Source: CAD feature listing. Evaluate the final solid. Frame: model axes, mm. Face numbers are marked on the shaded views. Give positions to 0.01 mm unless a question says otherwise; leave off trailing zeros. Loops run counter-clockwise (first coordinate to the right, second up) from the corner with the lowest first, then second, coordinate; pieces in that order, holes last. Notation, with made-up numbers: (5.25, 43.5) -> (62.25, 43.5) arc R16 cw to (62.25, 54.5) -> close; hole circle Ø10 at (82, 77). An arc over 180 degrees is marked (long way). Return JSON: item names as keys, results as strings. Group by question number.
(1) Pin query (flat end, axial travel): pin 1 (10 mm diameter, centred on x = 5.5, y = 67, fed in from -Z); pin 2 (4 mm diameter, centred on x = 5.5, y = 5.58, fed in from +Z); pin 3 (5 mm diameter, centred on x = 11, y = 56.8, fed in from +Z). Return the tip coordinate at first contact, or that it passes through.
(2) Draft query along X for the marked faces 1, 2 and 3. Return one class per face: released by +X, released by -X, zero draft, split by the parting line, or undercut.
(3) Ray query, line 1 (Y direction, x = 31, z = 4); line 2 (X direction, y = 56.8, z = 1.3); line 3 (Y direction, x = 31, z = 1). Return the intervals inside material, ascending. Write a range as from..to.
(4) Cut plane D-D on z = 4.2. Give the number of separate pieces and of enclosed holes in the cut face, then the cut area to 3 significant figures.
(5) Cut plane C-C on x = 11. Return loops of the section in (y, z).
(6) Cut plane B-B on y = 21.08. Return loops of the section in (x, z), then the cut area to 3 significant figures.
(7) Cut plane A-A on y = 36.58. Return loops of the section in (x, z) (3 decimals), then the cut area to 3 significant figures.
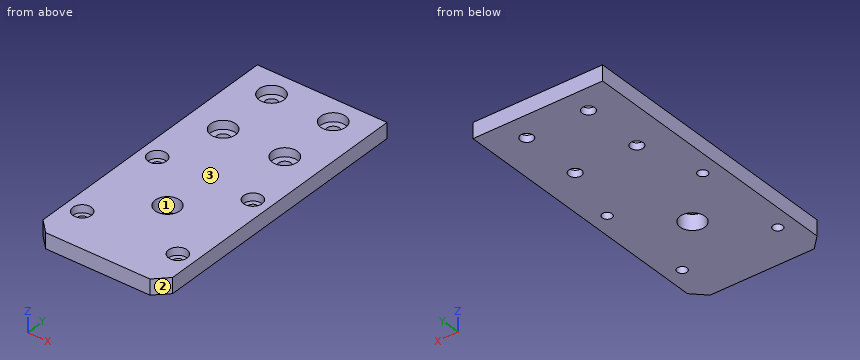
```python
from build123d import *

# Parameters (mm, degrees)
CROQUIS1_W              = 42
CROQUIS1_H              = 85
CROQUIS1_R              = 2.05
SALIENTE_EXTRUIR1_DEPTH = 5
CROQUIS4_R              = 4.05
CORTAR_EXTRUIR1_DEPTH   = 2.8
CROQUIS5_R              = 1.575
CROQUIS5_R_2            = 4
CORTAR_EXTRUIR2_DEPTH   = 6
CROQUIS6_R              = 3
CORTAR_EXTRUIR3_DEPTH   = 2.5
CROQUIS7_W              = 42
CROQUIS7_H              = 7.7
SALIENTE_EXTRUIR2_DEPTH = 5
CHAFL_N1_SIZE           = 4.1


with BuildPart() as part:
    # Croquis1 → Saliente-Extruir1 (new body)
    with BuildSketch(Plane.XY):
        with Locations((21, 42.5)):
            Rectangle(CROQUIS1_W, CROQUIS1_H)
        with Locations((11, 76.8)):
            Circle(CROQUIS1_R, mode=Mode.SUBTRACT)
        with Locations((31, 76.8)):
            Circle(CROQUIS1_R, mode=Mode.SUBTRACT)
        with Locations((31, 56.8)):
            Circle(CROQUIS1_R, mode=Mode.SUBTRACT)
        with Locations((11, 56.8)):
            Circle(CROQUIS1_R, mode=Mode.SUBTRACT)
    extrude(amount=SALIENTE_EXTRUIR1_DEPTH)

    # Croquis4 → Cortar-Extruir1 (cut)
    with BuildSketch(Plane.XY.offset(5)):
        with Locations((11, 76.8)):
            Circle(CROQUIS4_R)
        with Locations((11, 56.8)):
            Circle(CROQUIS4_R)
        with Locations((31, 56.8)):
            Circle(CROQUIS4_R)
        with Locations((31, 76.8)):
            Circle(CROQUIS4_R)
    extrude(amount=-CORTAR_EXTRUIR1_DEPTH, mode=Mode.SUBTRACT)

    # Croquis5 → Cortar-Extruir2 (cut, through all)
    with BuildSketch(Plane.XY.offset(5)):
        with Locations((5.5, 36.58)):
            Circle(CROQUIS5_R)
        with Locations((36.5, 36.58)):
            Circle(CROQUIS5_R)
        with Locations((36.5, 5.58)):
            Circle(CROQUIS5_R)
        with Locations((5.5, 5.58)):
            Circle(CROQUIS5_R)
        with Locations((21, 21.08)):
            Circle(CROQUIS5_R_2)
    extrude(amount=-CORTAR_EXTRUIR2_DEPTH, mode=Mode.SUBTRACT)

    # Croquis6 → Cortar-Extruir3 (cut)
    with BuildSketch(Plane.XY.offset(5)):
        with Locations((5.5, 36.58)):
            Circle(CROQUIS6_R)
        with Locations((36.5, 36.58)):
            Circle(CROQUIS6_R)
        with Locations((36.5, 5.58)):
            Circle(CROQUIS6_R)
        with Locations((5.5, 5.58)):
            Circle(CROQUIS6_R)
    extrude(amount=-CORTAR_EXTRUIR3_DEPTH, mode=Mode.SUBTRACT)

    # Croquis7 → Saliente-Extruir2 (add, through all)
    with BuildSketch(Plane(origin=(0, 0, 0), x_dir=(-1, 0, 0), z_dir=(0, 0, -1))):
        with Locations((-21, -3.85)):
            Rectangle(CROQUIS7_W, CROQUIS7_H)
    extrude(amount=-SALIENTE_EXTRUIR2_DEPTH)

    # Chaflán1
    chafl_n1_edges = [part.edges().sort_by_distance(p)[0] for p in [
        (42, -7.7, 2.5),
        (0, -7.7, 2.5),
    ]]
    chamfer(chafl_n1_edges, length=CHAFL_N1_SIZE)


solid = part.part
```
Answers:
{
 "1": {"pin 1": "z = 0", "pin 2": "z = 2.5", "pin 3": "z = 2.2"},
 "2": {"face 1": "undercut", "face 2": "released by +X", "face 3": "zero draft"},
 "3": {"line 1": "-7.7..52.75, 60.85..72.75, 80.85..85", "line 2": "0..8.95, 13.05..28.95, 33.05..42", "line 3": "-7.7..54.75, 58.85..74.75, 78.85..85"},
 "4": {"separate pieces": "1", "enclosed holes": "9", "area": "3,510 mm²"},
 "5": {"outline": "(-7.7, 0) -> (54.75, 0) -> (54.75, 2.2) -> (52.75, 2.2) -> (52.75, 5) -> (-7.7, 5) -> close; (58.85, 0) -> (74.75, 0) -> (74.75, 2.2) -> (72.75, 2.2) -> (72.75, 5) -> (60.85, 5) -> (60.85, 2.2) -> (58.85, 2.2) -> close; (78.85, 0) -> (85, 0) -> (85, 5) -> (80.85, 5) -> (80.85, 2.2) -> (78.85, 2.2) -> close"},
 "6": {"outline": "(0, 0) -> (17, 0) -> (17, 5) -> (0, 5) -> close; (25, 0) -> (42, 0) -> (42, 5) -> (25, 5) -> close", "area": "170 mm²"},
 "7": {"outline": "(0, 0) -> (3.925, 0) -> (3.925, 2.5) -> (2.5, 2.5) -> (2.5, 5) -> (0, 5) -> close; (7.075, 0) -> (34.925, 0) -> (34.925, 2.5) -> (33.5, 2.5) -> (33.5, 5) -> (8.5, 5) -> (8.5, 2.5) -> (7.075, 2.5) -> close; (38.075, 0) -> (42, 0) -> (42, 5) -> (39.5, 5) -> (39.5, 2.5) -> (38.075, 2.5) -> close", "area": "164 mm²"}
}
